Build history of the part. All positions in model axes, mm. A direction names the side the tool comes from. Coordinates: 2 decimals unless noted, no trailing zeros. Write each loop counter-clockwise with the first axis right and the second up, starting at its lowest first coordinate (ties: lowest second). Pieces come first, ordered by that corner, then holes. Notation, with made-up numbers: (-1, 82.25) -> (32, 82.25) arc R6 ccw to (32, 89.25) -> close; hole circle Ø6 at (-38.5, 73.5). An arc over 180 degrees is marked (long way). Write each question's results on one line, items separated by ' | '. Start each with the question number.
Q1. Saw through at A-A on y = 234.5. Give the cut face in (x, z), and give its area (3 significant figures).
Q2. Tool access for faces 1 (the face through (-1, 609.6, -15)), 2 (the face through (1, -9, 0)): list every direction of +Z, -Z, +X, -X, +Y, -Y with a clear straight run to the whole face (end or side of a thin tool).
Q3. Saw through at C-C on x = 30. Give the cut face in (y, z), and give its area (3 significant figures).
Q4. Drop flat-ended pins along their axis: pin 1 Ø10 at (x, y) = (-45, 452) entering from -Z; pin 2 Ø8.5 at (x, z) = (-19, -35.5) entering from +Y; pin 3 Ø10 at (y, z) = (282.5, -16.5) entering from -X. Give the stop position or say it passes through.
Q5. Two-plate mould, pull along Y, no slides. Class faces 3 (the face through (-24.1, -8.5, -46.8)), 4 (the face through (-1, -612.648, -15)), 5 (the face through (-55.335, -8.577, -15.027)): released by +Y, released by -Y, zero draft, split by the parting line, or undercut.
Q6. Saw through at B-B on z = -20.5. Give the cut face in (x, y).
Q7. Drill centre lines: line 1 (Z direction, x = 26.5, y = -369.5); line 2 (Z direction, x = -24.5, y = 104); line 3 (Y direction, x = -11, z = -10.5). Where is each one in solid material? Low to high.
from build123d import *

# Parameters (mm, degrees)
F1_DEPTH = 609.6
F0_R     = 19.05
F4_DEPTH = 3.048


with BuildPart() as f1:
    # F0 (on Front) → F1 (new body, symmetric)
    with BuildSketch(Plane.XZ):
        Polygon((49.8661872596, 0), (0, 0), (0, -6.096), (45.9889498077, -6.096), (54.864, -30.48), (60.96, -30.48), align=None)
    extrude(amount=F1_DEPTH, both=True)



with BuildPart() as f1b:
    # F0 (on Front) → F1, piece 2 (new body, symmetric)
    with BuildSketch(Plane.XZ):
        with Locations((28.194, -28.194)):
            Circle(F0_R)
    extrude(amount=F1_DEPTH, both=True)


with BuildPart() as f1_1:
    add(f1.part)
    # F2: F1b, F1 across plane
    add(f1b.part.mirror(Plane.YZ))
    add(f1.part.mirror(Plane.YZ))


    add(f1b.part)  # F4 merges F1b
    # F3 (on face) → F4 (join)
    with BuildSketch(Plane.XZ.offset(609.6)):
        Polygon((49.8661872596, 0), (-49.8661872596, 0), (-60.96, -30.48), (60.96, -30.48), align=None)
    extrude(amount=F4_DEPTH)

    # F5: F1 across plane


with BuildPart() as f1_2:
    add(f1_1.part)
    add(f1_1.part.mirror(Plane.XZ))


solid = f1_2.part
Returned:
1) outline: (-60.96, -30.48) -> (-54.86, -30.48) -> (-45.99, -6.1) -> (45.99, -6.1) -> (54.86, -30.48) -> (60.96, -30.48) -> (49.87, 0) -> (-49.87, 0) -> close; circle Ø38.1 at (-28.19, -28.19); circle Ø38.1 at (28.19, -28.19) | area: 3,200 mm2
2) face 1: none | face 2: +Z, +X, -X, +Y, -Y
3) outline: (-612.65, -30.48) -> (-609.6, -30.48) -> (-609.6, -47.16) -> (609.6, -47.16) -> (609.6, -30.48) -> (612.65, -30.48) -> (612.65, 0) -> (-612.65, 0) -> close; hole (-609.6, -9.23) -> (609.6, -9.23) -> (609.6, -6.1) -> (-609.6, -6.1) -> close | area: 53,900 mm2
4) pin 1: stops at z = -43.14 | pin 2: stops at y = 609.6 | pin 3: stops at x = -57.69
5) face 3: undercut | face 4: released by -Y | face 5: zero draft
6) outline: (-57.33, -612.65) -> (57.33, -612.65) -> (57.33, 612.65) -> (-57.33, 612.65) -> close; hole (-51.23, -609.6) -> (-45.62, -609.6) -> (-45.62, 609.6) -> (-51.23, 609.6) -> close; hole (-10.77, -609.6) -> (10.77, -609.6) -> (10.77, 609.6) -> (-10.77, 609.6) -> close; hole (45.62, -609.6) -> (51.23, -609.6) -> (51.23, 609.6) -> (45.62, 609.6) -> close
7) line 1: z = -47.17 to -9.22, -6.1 to 0 | line 2: z = -46.88 to -9.51, -6.1 to 0 | line 3: y = -612.65 to -609.6, 609.6 to 612.65
